Verification items for this drawing (mm, ordinates from the low corner). Round coordinates to 2 decimals unless told otherwise and drop trailing zeros. Loops run counter-clockwise (first coordinate to the right, second up) from the corner with the lowest first, then second, coordinate; pieces in that order, holes last. Notation, with made-up numbers: (-19, 29) - (-1, 29) arc R22 ccw to (-1, 63) - close; hole circle Ø4 at (-37.75, 78.5). An arc over 180 degrees is marked (long way). Put each result on its own line as item: value.
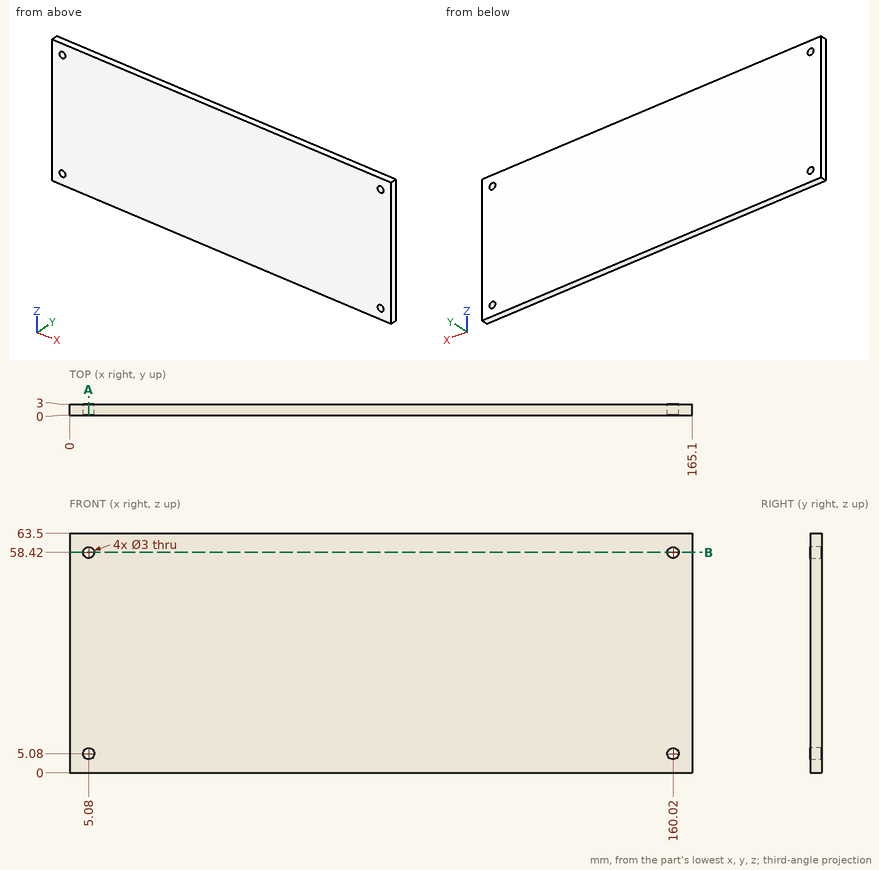
Item 1: Section check A-A on x = 5.08. Enter the section's corners in (y, z), then the cut area to 4 significant figures.
Filled sheet:
outline: (0, 0) - (3, 0) - (3, 3.58) - (0, 3.58) - close; (0, 6.58) - (3, 6.58) - (3, 56.92) - (0, 56.92) - close; (0, 59.92) - (3, 59.92) - (3, 63.5) - (0, 63.5) - close
area: 172.5 mm²
Item 2: Section check B-B on z = 58.42. Enter the section's corners in (x, y), then the cut area to 3 significant figures.
Filled sheet:
outline: (0, 0) - (3.58, 0) - (3.58, 3) - (0, 3) - close; (6.58, 0) - (158.52, 0) - (158.52, 3) - (6.58, 3) - close; (161.52, 0) - (165.1, 0) - (165.1, 3) - (161.52, 3) - close
area: 477 mm²
Item 3: Thickness scan on line 1 (Z direction, x = 160.02, y = 1.85); line 2 (X direction, y = 1.05, z = 5.08); line 3 (X direction, y = 2.65, z = 4.5). Record the ranges inside material, lowest first. Write a range as from..to.
Filled sheet:
line 1: 0..3.58, 6.58..56.92, 59.92..63.5
line 2: 0..3.58, 6.58..158.52, 161.52..165.1
line 3: 0..3.7, 6.46..158.64, 161.4..165.1
